```python
from build123d import *

# Parameters (mm, degrees)
BOSS_EXTRUDE1_DEPTH     = 60
SKETCH2_W               = 8
SKETCH2_H               = 10
BOSS_EXTRUDE3_DEPTH     = 60
SKETCH3_R               = 1.5
CUT_EXTRUDE1_DEPTH      = 60
FILLET1_R               = 4
CUT_EXTRUDE2_DEPTH      = 60
CUT_EXTRUDE2_DEPTH_BACK = 60
FILLET3_R               = 1
SKETCH5_R               = 2.607227144
BOSS_EXTRUDE4_DEPTH     = 5


with BuildPart() as part:
    # Sketch1 → Boss-Extrude1 (new body)
    with BuildSketch(Plane(origin=(0, 0, 0), x_dir=(1, 0, 0), z_dir=(0, 1, 0))):
        Polygon((4, 0), (-4, 0), (-4, -10), (-7.150933922, -14.5), (-4, -14.5), (4, -14.5), (7.150933922, -14.5), (4, -10), align=None)
    extrude(amount=BOSS_EXTRUDE1_DEPTH)

    # Sketch2 → Boss-Extrude3 (add)
    with BuildSketch(Plane(origin=(0, 0, 0), x_dir=(1, 0, 0), z_dir=(0, 1, 0))):
        with Locations((0, 5)):
            Rectangle(SKETCH2_W, SKETCH2_H)
    extrude(amount=BOSS_EXTRUDE3_DEPTH)

    # Sketch3 → Cut-Extrude1 (cut)
    with BuildSketch(Plane(origin=(0, 0, 0), x_dir=(1, 0, 0), z_dir=(0, 1, 0))):
        with Locations(Location((0, 6, 0), (0, 0, 270))):
            Circle(SKETCH3_R)
    extrude(amount=CUT_EXTRUDE1_DEPTH, mode=Mode.SUBTRACT)

    # Fillet1
    fillet1_edges = [part.edges().sort_by_distance(p)[0] for p in [
        (-4, 30, -10),
        (4, 30, -10),
    ]]
    fillet(fillet1_edges, radius=FILLET1_R - 0.0001)  # a hair under: the kernel refuses the full size

    # Sketch4 → Cut-Extrude2 (cut, two sides: drawn at the far end of the back side and taken through both)
    with BuildSketch(Plane(origin=(0, 0, 0), x_dir=(0, 0, -1), z_dir=(1, 0, 0)).offset(-CUT_EXTRUDE2_DEPTH_BACK)):
        Polygon((12.627548849, 60), (16.888144273, 60), (16.888144273, 0), (13.444072136, 0), (13.444072136, 10), (2, 10), (2, 15), (13.444072136, 15), (13.444072136, 20), (2, 20), (2, 25), (13.444072136, 25), (13.444072136, 30), (2, 30), (2, 35), (13.444072136, 35), (13.444072136, 40), (2, 40), (2, 45), (2, 50), (12.627548849, 50), align=None)
    extrude(amount=CUT_EXTRUDE2_DEPTH + CUT_EXTRUDE2_DEPTH_BACK, mode=Mode.SUBTRACT)

    # Fillet3
    fillet3_edges = [part.edges().sort_by_distance(p)[0] for p in [
        (-4, 12.5, -2),
        (4, 12.5, -2),
        (4, 22.5, -2),
        (4, 32.5, -2),
        (4, 45, -2),
        (-4, 45, -2),
        (-4, 32.5, -2),
        (-4, 22.5, -2),
    ]]
    fillet(fillet3_edges, radius=FILLET3_R)

    # Sketch5 → Boss-Extrude4 (add)
    with BuildSketch(Plane(origin=(0, 0, 0), x_dir=(1, 0, 0), z_dir=(0, 1, 0))):
        with Locations((0, 6)):
            Circle(SKETCH5_R)
    extrude(amount=BOSS_EXTRUDE4_DEPTH)


solid = part.part
```
The listing builds one solid part. Answer for the finished solid, in the listing's coordinates (mm). A direction names the side the tool comes from. Coordinates: 2 decimals unless noted, no trailing zeros. Loops run counter-clockwise (first coordinate to the right, second up) from the corner with the lowest first, then second, coordinate; pieces in that order, holes last. Notation, with made-up numbers: (-28, 87.25) - (-24, 87.25) arc R22 ccw to (-24, 118.25) - close; hole circle Ø7 at (-8.5, -15.5). An arc over 180 degrees is marked (long way). Use a Markdown table: item, result. Add a question column.
1) The part is cut by section B-B, the plane y = 43.5. Give the vertices of the cut face in (x, z).
2) Given pin 1 (5 mm diameter, centred on x = 0, y = 47, fed in from -Z); pin 2 (1 mm diameter, centred on y = 50, z = 11.5, fed in from +X); pin 3 (2 mm diameter, centred on y = 34.5, z = 7.5, fed in from +X), each flat-ended and moving along its own axis, determine where each tip first touches the part or whether it passes through.
3) Find the intervals of material crossed by line 1 (X direction, y = 54, z = -6); line 2 (Z direction, x = 0, y = 56); line 3 (Z direction, x = 2.5, y = 46), in increasing order.
4) The part is cut by section C-C, the plane z = 8.75. Give the vertices of the cut face in (x, y).
5) The part is cut by section D-D, the plane z = 11.25. Give the vertices of the cut face in (x, y).
6) For faces 4 (the flat face through (0, 12, -2)), 5 (the flat face through (4, 30, 2)), 6 (the cylindrical face through (3.699, 12.535, -1.715)), 7 (the cylindrical face through (0.07, 37.47, -7.5)), 8 (the cylindrical face through (-2.859, 27.535, -8.797)), determine the directions among +Z, -Z, +X, -X, +Y, -Y from which every point of the face is accessible in a straight line to the end or side of a thin tool.
7) The mould has two halves that part along Z. Classify faces 1 (the cylindrical face through (-2.859, 37.535, -8.797)), 2 (the flat face through (-4, 30, 2)), 3 (the cylindrical face through (0.07, 7.46, -7.5)): released by +Z, released by -Z, zero draft, split by the parting line, or undercut.
Here are the results:
| question | item | result |
|---|---|---|
| 1 | outline | (-7.15, 14.5) - (-4, 10) - (-4, -1) arc R1 ccw to (-3, -2) - (3, -2) arc R1 ccw to (4, -1) - (4, 10) - (7.15, 14.5) - close |
| 2 | pin 1 | stops at z = -2 |
| 2 | pin 2 | stops at x = 5.4 |
| 2 | pin 3 | stops at x = 4 |
| 3 | line 1 | x = -4 to -1.5, 1.5 to 4 |
| 3 | line 2 | z = -10 to -7.5, -4.5 to 14.5 |
| 3 | line 3 | z = -2 to 14.5 |
| 4 | outline | (-4, 0) - (4, 0) - (4, 60) - (-4, 60) - close |
| 5 | outline | (-4.88, 0) - (4.88, 0) - (4.88, 60) - (-4.88, 60) - close |
| 6 | face 4 | -Z, +X, -X |
| 6 | face 5 | -Z, +X, +Y, -Y |
| 6 | face 6 | -Z, +X |
| 6 | face 7 | +Y |
| 6 | face 8 | -Z, -X, +Y, -Y |
| 7 | face 1 | released by -Z |
| 7 | face 2 | zero draft |
| 7 | face 3 | undercut |
